Source: three-view drawing plus pictorial views. Frame: mm from the lowest corner of the part. Give positions to 0.01 mm unless a question says otherwise; leave off trailing zeros. Write each loop counter-clockwise with the first axis right and the second up, starting at its lowest first coordinate (ties: lowest second). Pieces come first, ordered by that corner, then holes.
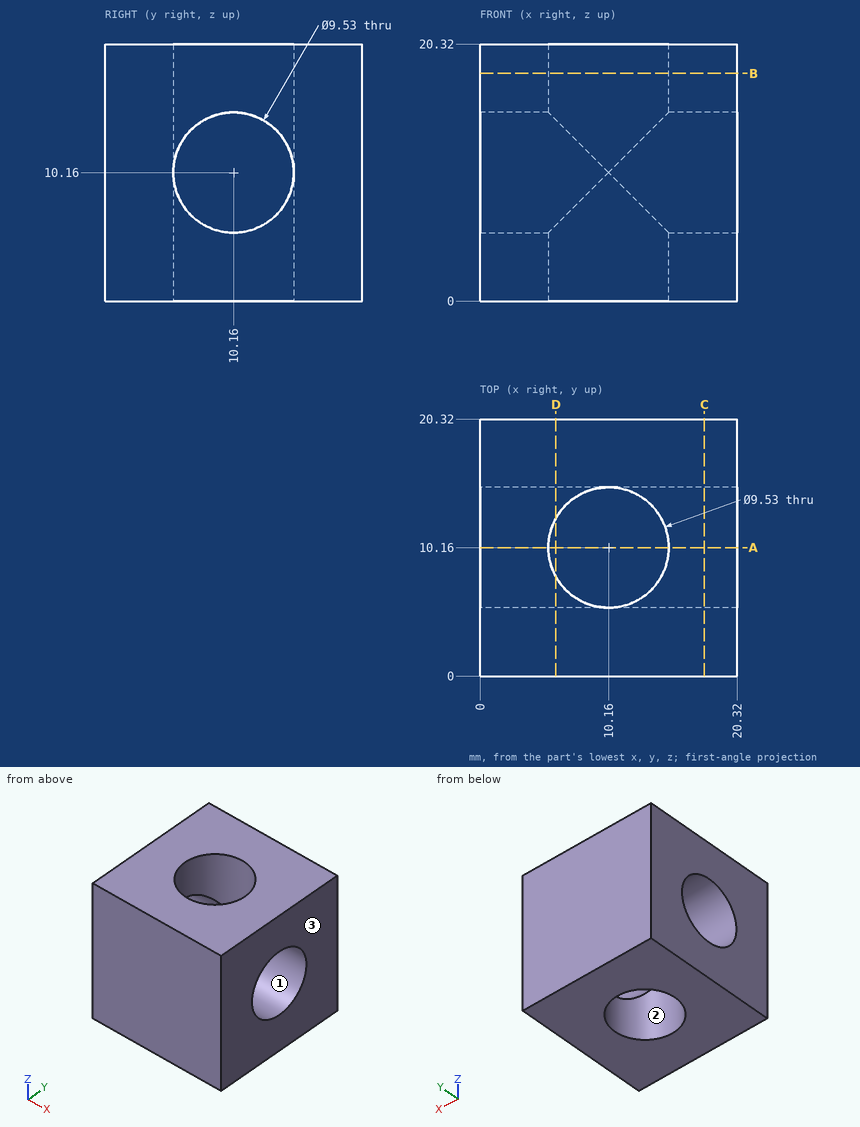
Q1. Section B-B on z = 18. Output: boundary loops of the cut face in (x, y) (3 decimals).
Filled sheet:
outline: (0, 0) - (20.32, 0) - (20.32, 20.32) - (0, 20.32) - close; hole circle Ø9.53 at (10.16, 10.16)
Q2. Section A-A on y = 10.16. Output: boundary loops of the cut face in (x, z) (3 decimals).
Filled sheet:
outline: (0, 0) - (5.395, 0) - (5.395, 5.395) - (0, 5.395) - close; (0, 14.925) - (5.395, 14.925) - (5.395, 20.32) - (0, 20.32) - close; (14.925, 0) - (20.32, 0) - (20.32, 5.395) - (14.925, 5.395) - close; (14.925, 14.925) - (20.32, 14.925) - (20.32, 20.32) - (14.925, 20.32) - close
Q3. Ray query, line 1 along X through (y, z) = (10.16, 4.75) (3 decimals). Return the intervals inside material, ascending.
Filled sheet:
line 1: x = 0 to 5.395, 14.925 to 20.32
Q4. Pull-direction query (X, two-part tool) for the marked faces 1, 2 and 3; classes: released by +X, released by -X, zero draft, split by the parting line, or undercut.
Filled sheet:
face 1: zero draft
face 2: undercut
face 3: released by +X
Q5. Section D-D on x = 6. Output: boundary loops of the cut face in (y, z) (3 decimals).
Filled sheet:
outline: (0, 0) - (7.836, 0) - (7.836, 6) arc R4.765 cw to (7.836, 14.32) - (7.836, 20.32) - (0, 20.32) - close; (12.484, 0) - (20.32, 0) - (20.32, 20.32) - (12.484, 20.32) - (12.484, 14.32) arc R4.765 cw to (12.484, 6) - close
